Geometry check sheet. Reference: the model listing, model coordinates, mm. Face numbers are marked on the shaded views. A direction names the side the tool comes from. Round coordinates to 2 decimals unless told otherwise and drop trailing zeros. Write each loop counter-clockwise with the first axis right and the second up, starting at its lowest first coordinate (ties: lowest second). Pieces come first, ordered by that corner, then holes. Notation, with made-up numbers: (-38, 52.25) - (-25, 52.25) arc R24 ccw to (-25, 74.25) - close; hole circle Ø8 at (-5, 1.5). An arc over 180 degrees is marked (long way). Return JSON: item names as keys, results as strings.
Autodesk Inventor part; units mm, degrees
ref_plane "YZ Plane" through (0, 0, 0) normal (1, 0, 0) x (0, 1, 0)
ref_plane "XZ Plane" through (0, 0, 0) normal (0, 1, 0) x (-1, 0, 0)
ref_plane "XY Plane" through (0, 0, 0) normal (0, 0, 1) x (1, 0, 0)
sketch "Sketch1" plane through (0, 0, 0) normal (0, 0, 1) x (1, 0, 0)
  point P0 (0, 0)
sketch "Sketch2" plane through (0, 0, 0) normal (0, 0, 1) x (1, 0, 0)
  line L0 (0, 0) -> (-50, 0)
  line L1 (0, 0) -> (-50, 0)
  line L2 (0, 0) -> (-50, 0)
  line L3 (-50, 0) -> (-50, 50)
  line L4 (-50, 50) -> (0, 50)
  line L5 (0, 50) -> (0, 0)
  line L6 (-31.5, 44) -> (-18.5, 44)
  line L7 (-18.5, 44) -> (-18.5, 21)
  line L8 (-18.5, 21) -> (-31.5, 21)
  line L9 (-31.5, 21) -> (-31.5, 44)
  circle A0 centre (-25, 46.8) radius 0.75
  circle A1 centre (-25, 18.2) radius 0.75
  line L10 (-37.5, 50) -> (-12.5, 50)
  line L11 (-12.5, 50) -> (-12.5, 10)
  line L12 (-12.5, 10) -> (-37.5, 10)
  line L13 (-37.5, 10) -> (-37.5, 50)
  line L14 (-37.5, 44) -> (-50, 44)
  line L15 (-12.5, 44) -> (0, 44)
  dimension "d4" = 50
  dimension "d5" = 50
  dimension "d6" = 13
  dimension "d7" = 23
  dimension "d8" = 18.5
  dimension "d9" = 6
  dimension "d10" = 1.5
  dimension "d11" = 6.5
  dimension "d12" = 2.8
  dimension "d13" = 1.5
  dimension "d14" = 6.5
  dimension "d15" = 2.8
  dimension "d16" = 25
  dimension "d17" = 40
  dimension "d18" = 12.5
extrude "Extrusion1" add sketch "Sketch2" along normal blind 20 contours L11 L12 L13 L4
extrude "Extrusion2" add sketch "Sketch2" along normal blind 3 contours L6 L7 L8 L9
extrude "Extrusion3" add sketch "Sketch2" against normal blind 3 contours L0 L3 L14 L13 L12 L11 L15 L5 | L15 L11 L4 L5 | L3 L4 L13 L14
extrude "Extrusion4" add sketch "Sketch2" against normal blind 3 contours L11 L12 L13 L4
extrude "Extrusion5" add sketch "Sketch2" against normal blind 3 contours L6 L7 L8 L9
sketch "Sketch3" plane through (-18.5, 21, 20) normal (-1, 0, 0) x (0, 0, 1)
  point P0 (-20, -21)
sketch "Sketch4" plane through (0, 0, -3) normal (0, 0, -1) x (-1, 0, 0)
  line L0 (12.5, 50) -> (37.5, 50)
  line L1 (37.5, 50) -> (37.5, 10)
  line L2 (12.5, 50) -> (37.5, 50)
  line L3 (37.5, 50) -> (37.5, 35.8782)
  line L4 (37.5, 35.8782) -> (12.5, 35.8782)
  line L5 (12.5, 35.8782) -> (12.5, 50)
  point P0 (0, 0)
extrude "Extrusion6" add sketch "Sketch4" along normal blind 40
sketch "Sketch5" plane through (-37.5, 35.8782, -3) normal (0, -1, 0) x (1, 0, 0)
  line L0 (0, -40) -> (25, -40)
  line L1 (25, -40) -> (0, -40)
  line L2 (0, -40) -> (0, -28)
  line L3 (0, -28) -> (25, -28)
  line L4 (25, -28) -> (25, -40)
  point P0 (37.5, 3)
  dimension "d31" = 25
  dimension "d32" = 12
extrude "Extrusion7" add sketch "Sketch5" along normal blind 30
sketch "Sketch6" plane through (0, 0, -43) normal (0, 0, -1) x (-1, 0, 0)
  circle A0 centre (25, 22) radius 5.4
  line L0 (37.5, 50) -> (12.5, 50)
  line L1 (37.5, 50) -> (37.5, 5.8782)
  point P0 (0, 0)
  dimension "d35" = 10.8
  dimension "d36" = 28
  dimension "d37" = 12.5
hole "Hole1" at (-25, 22, -43) direction (0, 0, 1) diameter 10.8 depth 12
sketch "Sketch7" plane through (-37.5, 50, 20) normal (0, 1, 0) x (1, 0, 0)
  line L0 (0, 20) -> (25, 20)
  line L1 (7.5, 20) -> (17.5, 20)
  line L2 (17.5, 20) -> (17.5, 15)
  line L3 (17.5, 15) -> (7.5, 15)
  line L4 (7.5, 15) -> (7.5, 20)
  line L5 (0, 20) -> (0, 0)
  point P0 (37.5, 20)
  dimension "d47" = 10
  dimension "d48" = 5
  dimension "d49" = 7.5
extrude "Extrusion8" cut sketch "Sketch7" against normal blind 10
extrude "Extrusion9" cut sketch "Sketch2" against normal blind 2 contours L6 L7 L8 L9
extrude "Extrusion10" cut sketch "Sketch2" along normal blind 3 contours L6 L7 L8 L9
extrude "Extrusion11" add sketch "Sketch2" against normal blind 3 contours L6 L7 L8 L9
extrude "Extrusion12" cut sketch "Sketch2" against normal blind 4 contours L6 L7 L8 L9
thicken "Thicken1" operation add thickness 12.5 both sides no extend neighbours yes toward (1, 0, 0) faces at (-12.5, 45.2927, -25.6667)
thicken "Thicken2" operation add thickness 12.5 both sides no extend neighbours yes toward (-1, 0, 0) faces at (-37.5, 45.2927, -25.6667)
thicken "Thicken3" operation add thickness 0.5 both sides no extend neighbours yes toward (0, -1, 0) faces at (-27.1667, 21, 12.3333)
thicken "Thicken4" operation add thickness 0.5 both sides no extend neighbours yes toward (0, 1, 0) faces at (-26.6667, 44, 15)
sketch "Sketch8" plane through (0, 5.8782, -31) normal (0, 0, 1) x (1, 0, 0)
  point P0 (0, -5.8782)
sketch "Sketch9" plane through (0, 5.8782, -31) normal (0, 0, 1) x (1, 0, 0)
  circle A0 centre (-25, 16.1218) radius 5.4
  circle A1 centre (-25, 16.1218) radius 9.9
  line L0 (-25, 6.2218) -> (-33.5737, 11.1718)
  line L1 (-33.5737, 11.1718) -> (-33.5737, 21.0718)
  line L2 (-33.5737, 21.0718) -> (-25, 26.0218)
  line L3 (-25, 26.0218) -> (-16.4263, 21.0718)
  line L4 (-16.4263, 21.0718) -> (-16.4263, 11.1718)
  line L5 (-16.4263, 11.1718) -> (-25, 6.2218)
  point P0 (0, -5.8782)
  dimension "d68" = 19.8
extrude "Extrusion13" cut sketch "Sketch9" against normal blind 6.8 contours A0 | L4 L5 L0 L1 L2 L3
thicken "Thicken5" operation add thickness 3.978 both sides no extend neighbours yes toward (0, -1, 0) faces at (-22.8333, 35.8782, -22)
thicken "Thicken6" operation add thickness 3 both sides no extend neighbours yes toward (0, 0, -1) faces at (-25, 42.4667, -43)
extrude "Extrusion14" add sketch "Sketch2" along normal up to surface (20 mm away) contours L15 L11 L4 L5 | L3 L4 L13 L14
sketch "Sketch10" plane through (-50, 44, 20) normal (0, -1, 0) x (1, 0, 0)
  point P0 (50, -20)
sketch "Sketch11" plane through (-50, 44, 20) normal (0, -1, 0) x (1, 0, 0)
  line L0 (12.5, -20) -> (0, 0)
  line L1 (12.5, 0) -> (12.5, -20)
  line L2 (12.5, 0) -> (0, -20)
  point P0 (50, -20)
  point P1 (6.25, -10)
hole "Hole2" at (-43.75, 44, 10) direction (0, 1, 0) diameter 4.3 end through all
sketch "Sketch12" plane through (-12.5, 44, 20) normal (0, -1, 0) x (1, 0, 0)
  line L0 (0, -20) -> (0, 0)
  line L1 (12.5, -20) -> (0, 0)
  line L2 (12.5, 0) -> (0, -20)
  point P0 (6.25, -10)
hole "Hole3" at (-6.25, 44, 10) direction (0, 1, 0) diameter 4.3 end through all
sketch "Sketch13" plane through (-50, 50, 20) normal (0, 1, 0) x (1, 0, 0)
  circle A0 centre (6.25, 10) radius 2.15
  circle A1 centre (6.25, 10) radius 2.15
  circle A2 centre (43.75, 10) radius 2.15
  circle A3 centre (43.75, 10) radius 2.15
  line L0 (-0.0918, 20) -> (50, 20)
  line L1 (50, 20) -> (50, 0)
  line L2 (50, 0) -> (-0.0918, 0)
  line L3 (-0.0918, 0) -> (-0.0918, 20)
properties part number "servo_holder"
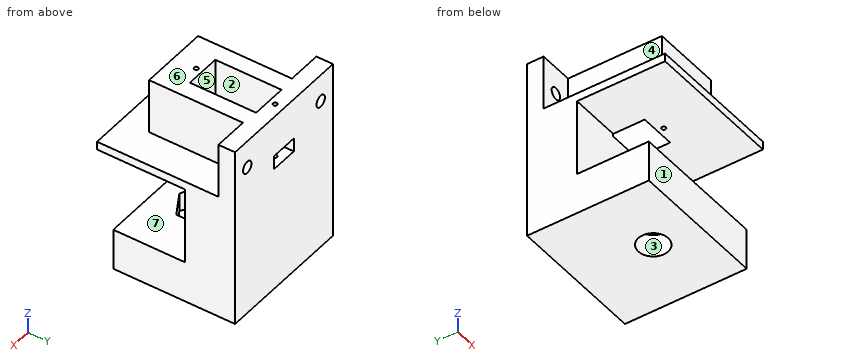
(1) Release check for a two-part mould opening along Z. For the marked faces 5, 6 and 7 record: pulls with the +Z half, pulls with the -Z half, needs draft (parallel to the pull), parting line crosses it, or undercut.
Response values:
{"face 5": "needs draft", "face 6": "pulls with the +Z half", "face 7": "undercut"}
(2) Section check D-D, the plane y = 41. Enter the section's corners in (x, z), plus the area to 3 significant figures.
Response values:
{"outline": "(-50, -46) - (0, -46) - (0, 0) - (-12.5, 0) - (-12.5, 20) - (-18.5, 20) - (-18.5, -4) - (-31.5, -4) - (-31.5, 20) - (-37.5, 20) - (-37.5, 0) - (-50, 0) - close", "area": "2,490 mm^2"}
(3) Access from +Z, -Z, +X, -X, +Y, -Y to the whole of each face (thin tool, end or side, straight path). Record for the marked faces 1, 2, 3 and 4.
Response values:
{"face 1": "-Z, +X, -X, -Y", "face 2": "+Z", "face 3": "-Z", "face 4": "+Z, -X, -Y"}
(4) Gauge pin test, flat ends, axial feed: pin 1 (22.5 mm diameter, centred on x = -25.5, z = -13, fed in from -Y); pin 2 (10 mm diameter, centred on y = 28, z = 9.5, fed in from -X); pin 3 (3 mm diameter, centred on x = -33.5, z = 11.5, fed in from -Y); pin 4 (6 mm diameter, centred on x = -43.5, z = 12.5, fed in from -Y). Record the tip position at first contact, or that the pin passes through.
Response values:
{"pin 1": "stops at y = 0", "pin 2": "stops at x = -37.5", "pin 3": "stops at y = 10", "pin 4": "stops at y = 44"}
(5) Section check C-C, the plane x = -6.25. Enter the section's corners in (y, z), plus the area to 3 significant figures.
Response values:
{"outline": "(0, -3) - (31.9, -3) - (31.9, -31) - (5.88, -31) - (5.88, -46) - (50, -46) - (50, 7.85) - (44, 7.85) - (44, 0) - (0, 0) - close; (44, 12.15) - (50, 12.15) - (50, 20) - (44, 20) - close", "area": "1,410 mm^2"}
(6) Section check B-B, the plane y = 22. Enter the section's corners in (x, z).
Response values:
{"outline": "(-50, -46) - (-30.4, -46) - (-30.4, -37.8) - (-33.57, -37.8) - (-33.57, -31) - (-50, -31) - close; (-50, -3) - (-31.5, -3) - (-31.5, 20) - (-37.5, 20) - (-37.5, 0) - (-50, 0) - close; (-19.6, -46) - (0, -46) - (0, -31) - (-16.43, -31) - (-16.43, -37.8) - (-19.6, -37.8) - close; (-18.5, -3) - (0, -3) - (0, 0) - (-12.5, 0) - (-12.5, 20) - (-18.5, 20) - close"}
(7) Material ranges on line 1 along X through (y, z) = (32, 14.5); line 2 along Y through (x, z) = (-25, -1); line 3 along Z through (x, y) = (-40, 12), recorded low to high. Write a range as [from, to].
Response values:
{"line 1": "x = [-37.5, -31.5], [-18.5, -12.5]", "line 2": "y = [0, 17.45], [18.95, 20.5], [44.5, 46.05], [47.55, 50]", "line 3": "z = [-46, -31], [-3, 0]"}
(8) Section check A-A, the plane z = 10. Enter the section's corners in (x, y).
Response values:
{"outline": "(-50, 44) - (-45.9, 44) - (-45.9, 50) - (-50, 50) - close; (-41.6, 44) - (-37.5, 44) - (-37.5, 10) - (-12.5, 10) - (-12.5, 44) - (-8.4, 44) - (-8.4, 50) - (-41.6, 50) - close; (-4.1, 44) - (0, 44) - (0, 50) - (-4.1, 50) - close; hole (-31.5, 20.5) - (-18.5, 20.5) - (-18.5, 44.5) - (-31.5, 44.5) - close; hole circle Ø1.5 at (-25, 18.2); hole circle Ø1.5 at (-25, 46.8)"}
